Input: part model. Units: mm. Frame: model coordinates. Coordinates: 2 decimals unless noted, no trailing zeros. Order: outer loops, then holes, each group sorted by start corner. A loop starts at its lowest first (then second) coordinate and runs counter-clockwise, first axis right, second up. Notation, with made-up numbers: (87.5, -3.5) -> (118.5, -3.5) arc R16 cw to (118.5, 16.5) -> close; hole circle Ø7 at (-27.75, 0). An arc over 180 degrees is marked (long way). Answer as CSV lines item,"result".
from build123d import *

# Parameters (mm, degrees)
SALIENTE_EXTRUIR1_DEPTH = 540


with BuildPart() as part:
    # Croquis1 → Saliente-Extruir1 (new body)
    with BuildSketch(Plane.XY):
        with BuildLine():
            ThreePointArc((-13.23096405, 11.648445498), (-13.584517441, 11.501998889), (-13.73096405, 11.148445498))
            Line((-13.73096405, 11.148445498), (-13.73096405, 2.035658412))
            ThreePointArc((-13.73096405, 2.035658412), (-13.626281451, 1.729514406), (-13.356067441, 1.551562201))
            Line((-13.356067441, 1.551562201), (-12.169475815, 1.244915231))
            ThreePointArc((-12.169475815, 1.244915231), (-11.899261805, 1.066963026), (-11.794579206, 0.76081902))
            Line((-11.794579206, 0.76081902), (-11.794579206, 0.442917518))
            ThreePointArc((-11.794579206, 0.442917518), (-11.736179814, 0.265071669), (-11.583718232, 0.156466416))
            ThreePointArc((-11.583718232, 0.156466416), (-7.701884055, -0.773383829), (-3.73096405, -1.17965021))
            ThreePointArc((-3.73096405, -1.17965021), (0.239955955, -0.773383829), (4.121790132, 0.156466416))
            ThreePointArc((4.121790132, 0.156466416), (4.274251714, 0.265071669), (4.332651106, 0.442917518))
            Line((4.332651106, 0.442917518), (4.332651106, 0.76081902))
            ThreePointArc((4.332651106, 0.76081902), (4.437333704, 1.066963026), (4.707547715, 1.244915231))
            Line((4.707547715, 1.244915231), (5.894139341, 1.551562201))
            ThreePointArc((5.894139341, 1.551562201), (6.164353351, 1.729514406), (6.26903595, 2.035658412))
            Line((6.26903595, 2.035658412), (6.26903595, 11.148445498))
            ThreePointArc((6.26903595, 11.148445498), (6.12258934, 11.501998889), (5.76903595, 11.648445498))
            Line((5.76903595, 11.648445498), (3.76903595, 11.648445498))
            ThreePointArc((3.76903595, 11.648445498), (3.415482559, 11.501998889), (3.26903595, 11.148445498))
            Line((3.26903595, 11.148445498), (3.26903595, 10.648445498))
            ThreePointArc((3.26903595, 10.648445498), (-0.206558338, 10.028093004), (-3.73096405, 9.82034979))
            ThreePointArc((-3.73096405, 9.82034979), (-7.255369763, 10.028093004), (-10.73096405, 10.648445498))
            Line((-10.73096405, 10.648445498), (-10.73096405, 11.148445498))
            ThreePointArc((-10.73096405, 11.148445498), (-10.87741066, 11.501998889), (-11.23096405, 11.648445498))
            Line((-11.23096405, 11.648445498), (-13.23096405, 11.648445498))
        make_face()
    extrude(amount=SALIENTE_EXTRUIR1_DEPTH)


solid = part.part
1. Ray query, line 1 along Y through (x, z) = (3.5, 155); line 2 along Y through (x, z) = (-4.25, 203). Return the intervals inside material, ascending.
Findings:
line 1,"y = -0.03 to 11.57"
line 2,"y = -1.16 to 9.82"
2. Contact query for flat-ended pins moving along their axis: pin 1 (2 mm diameter, centred on x = -8, y = 0.5, fed in from -Z); pin 2 (6 mm diameter, centred on x = -3.5, z = 448.5, fed in from +Y). Output: stop coordinate, or through.
Findings:
pin 1,"stops at z = 0"
pin 2,"stops at y = 9.99"
3. Cut plane A-A (z = 231). Return the cut outline in (x, y), plus the area to 3 significant figures.
Findings:
outline,"(-13.73, 2.04) arc R0.5 ccw to (-13.36, 1.55) -> (-12.17, 1.24) arc R0.5 cw to (-11.79, 0.76) -> (-11.79, 0.44) arc R0.3 ccw to (-11.58, 0.16) arc R30 ccw to (-3.73, -1.18) arc R30 ccw to (4.12, 0.16) arc R0.3 ccw to (4.33, 0.44) -> (4.33, 0.76) arc R0.5 cw to (4.71, 1.24) -> (5.89, 1.55) arc R0.5 ccw to (6.27, 2.04) -> (6.27, 11.15) arc R0.5 ccw to (5.77, 11.65) -> (3.77, 11.65) arc R0.5 ccw to (3.27, 11.15) -> (3.27, 10.65) arc R30 cw to (-10.73, 10.65) -> (-10.73, 11.15) arc R0.5 ccw to (-11.23, 11.65) -> (-13.23, 11.65) arc R0.5 ccw to (-13.73, 11.15) -> close"
area,"216 mm2"
